Answer from the drawing. Dimensions are ordinates in mm from the lowest x, y and z of the part. Give positions to 0.01 mm unless a question says otherwise; leave off trailing zeros. Loops run counter-clockwise (first coordinate to the right, second up) from the corner with the lowest first, then second, coordinate; pieces in that order, holes last.
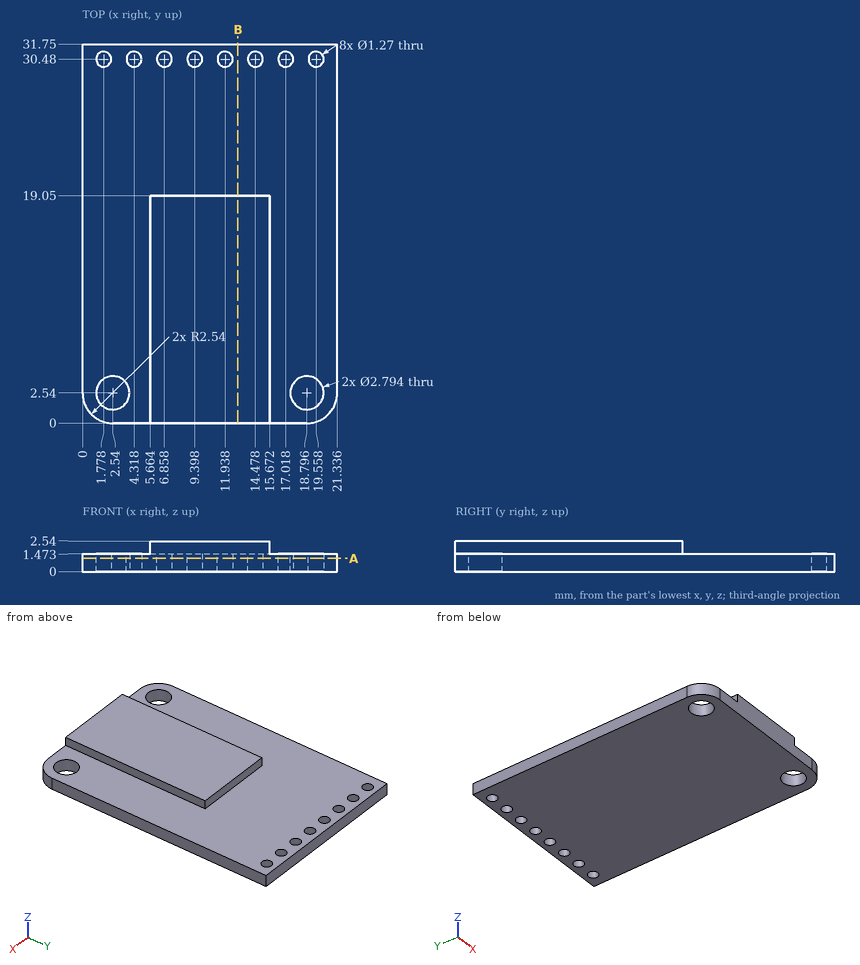
Item 1: Find section B-B, the plane x = 13. Write down the section's boundary in (y, z).
Item 2: Flat-ended cylindrical pins translate along their axes: pin 1 Ø1.5 at (x, y) = (9, 5.5) entering from -Z; pin 2 Ø2 at (x, y) = (11.938, 30.48) entering from +Z. Find the tip coordinate at first contact, or state that the pin passes through.
Item 3: Consider line 1 (Y direction, x = 2.5, z = 0.2); line 2 (Y direction, x = 19.5, z = 0.4); line 3 (Z direction, x = 20.5, y = 20.5). Determine where each line is inside the solid, lowest interval first.
Item 4: Find section A-A, the plane z = 1.1. Give the number of separate pieces and of enclosed holes in the cut face, plus the area to 3 significant figures.
Ans:
1. outline: (0, 0) - (31.75, 0) - (31.75, 1.47) - (19.05, 1.47) - (19.05, 2.54) - (0, 2.54) - close
2. pin 1: stops at z = 0
2. pin 2: stops at z = 1.47
3. line 1: y = 0 to 1.14, 3.94 to 31.75
3. line 2: y = 0.1 to 1.33, 3.75 to 29.85, 31.11 to 31.75
3. line 3: z = 0 to 1.47
4. separate pieces: 1
4. enclosed holes: 10
4. area: 652 mm2
